```python
from build123d import *

# Parameters (mm, degrees)
SKETCH1_W           = 51
SKETCH1_H           = 38.31
SKETCH1_R           = 8
BOSS_EXTRUDE1_DEPTH = 1.5875
SKETCH2_R           = 1.1303
CUT_EXTRUDE1_DEPTH  = 1.5875


with BuildPart() as part:
    # Sketch1 → Boss-Extrude1 (new body)
    with BuildSketch(Plane.XY):
        with Locations((25.5, 19.155)):
            Rectangle(SKETCH1_W, SKETCH1_H)
        with Locations((25.5, 19.155)):
            Circle(SKETCH1_R, mode=Mode.SUBTRACT)
    extrude(amount=BOSS_EXTRUDE1_DEPTH)

    # Sketch2 → Cut-Extrude1 (cut)
    with BuildSketch(Plane.XY.offset(1.5875)):
        with Locations((44, 35.31)):
            Circle(SKETCH2_R)
        with Locations((7, 35.31)):
            Circle(SKETCH2_R)
    extrude(amount=-CUT_EXTRUDE1_DEPTH, mode=Mode.SUBTRACT)


solid = part.part
```
Read the model definition and answer for the solid it produces. Units are mm, in the model's axes. Give positions to 0.01 mm unless a question says otherwise; leave off trailing zeros. Order: outer loops, then holes, each group sorted by start corner. A loop starts at its lowest first (then second) coordinate and runs counter-clockwise, first axis right, second up.
(1) Find section B-B (y = 35.31). Give the vertices of the cut face in (x, z), plus the area to 3 significant figures.
(2) Find section C-C (y = 20.5). Give the vertices of the cut face in (x, z).
(3) Given pin 1 (9.5 mm diameter, centred on x = 25.5, y = 19.155, fed in from +Z), flat-ended and moving along its own axis, determine where the tip first touches the part or whether it passes through.
(4) Find section D-D (z = 0.55). Give the vertices of the cut face in (x, y) (3 decimals).
(5) For a pull along X with two mould halves and no side action, classify faces 1 (the flat face through (25, 38.31, 1)), 2 (the cylindrical face through (6.85, 36.43, 0.8)), 3 (the flat face through (0, 19, 1)) as released by +X, released by -X, zero draft, split by the parting line, or undercut.
(6) Straight lines are drawn through the part: L1, parallel to Y at x = 44, z = 0.4; L2, parallel to Y at x = 25.5, z = 0.4 (3 decimals); L3, parallel to X at y = 24, z = 1.05. For each, find the intervals that lie inside material, in ascending order.
(7) Find section A-A (x = 25.5). Give the vertices of the cut face in (y, z) (1 decimal), plus the area to 3 significant figures.
Result sheet:
1. outline: (0, 0) - (5.87, 0) - (5.87, 1.59) - (0, 1.59) - close; (8.13, 0) - (42.87, 0) - (42.87, 1.59) - (8.13, 1.59) - close; (45.13, 0) - (51, 0) - (51, 1.59) - (45.13, 1.59) - close
1. area: 73.8 mm2
2. outline: (0, 0) - (17.61, 0) - (17.61, 1.59) - (0, 1.59) - close; (33.39, 0) - (51, 0) - (51, 1.59) - (33.39, 1.59) - close
3. pin 1: passes through
4. outline: (0, 0) - (51, 0) - (51, 38.31) - (0, 38.31) - close; hole circle Ø2.261 at (7, 35.31); hole circle Ø16 at (25.5, 19.155); hole circle Ø2.261 at (44, 35.31)
5. face 1: zero draft
5. face 2: undercut
5. face 3: released by -X
6. L1: y = 0 to 34.18, 36.44 to 38.31
6. L2: y = 0 to 11.155, 27.155 to 38.31
6. L3: x = 0 to 19.13, 31.87 to 51
7. outline: (0, 0) - (11.2, 0) - (11.2, 1.6) - (0, 1.6) - close; (27.2, 0) - (38.3, 0) - (38.3, 1.6) - (27.2, 1.6) - close
7. area: 35.4 mm2
